```python
from build123d import *

# Parameters (mm, degrees)
BOX138_W     = 17
BOX138_H     = 24
BOX138_DEPTH = 11
BOX137_W     = 43
BOX137_H     = 27
BOX137_DEPTH = 11
BOX136_W     = 50
BOX136_H     = 37
BOX136_DEPTH = 13
BOX135_W     = 55
BOX135_H     = 40
BOX135_DEPTH = 16


with BuildPart() as cube060:
    # Box138 → Box138 (new body)
    with BuildSketch(Plane(origin=(337.5, 106, 176), x_dir=(1, 0, 0), z_dir=(0, 0, -1))):
        with Locations((8.5, 12)):
            Rectangle(BOX138_W, BOX138_H)
    extrude(amount=BOX138_DEPTH)


with BuildPart() as cube059:
    # Box137 → Box137 (new body)
    with BuildSketch(Plane(origin=(345.5, 111, 185), x_dir=(1, 0, 0), z_dir=(0, 0, -1))):
        with Locations((21.5, 13.5)):
            Rectangle(BOX137_W, BOX137_H)
    extrude(amount=BOX137_DEPTH)


with BuildPart() as cube058:
    # Box136 → Box136 (new body)
    with BuildSketch(Plane(origin=(342, 121, 181.5), x_dir=(1, 0, 0), z_dir=(0, 0, -1))):
        with Locations((25, 18.5)):
            Rectangle(BOX136_W, BOX136_H)
    extrude(amount=BOX136_DEPTH)


with BuildPart() as cut026:
    # Box135 → Box135 (new body)
    with BuildSketch(Plane(origin=(340, 124, 183), x_dir=(1, 0, 0), z_dir=(0, 0, -1))):
        with Locations((27.5, 20)):
            Rectangle(BOX135_W, BOX135_H)
    extrude(amount=BOX135_DEPTH)

    # Cut024: cut Cube058
    add(cube058.part, mode=Mode.SUBTRACT)

    # Cut025: cut Cube059
    add(cube059.part, mode=Mode.SUBTRACT)

    # Cut026: cut Cube060
    add(cube060.part, mode=Mode.SUBTRACT)


solid = cut026.part
```
Model file for the job. Use its own axes, mm. A direction names the side the tool comes from. Round coordinates to 2 decimals unless told otherwise and drop trailing zeros. Write each loop counter-clockwise with the first axis right and the second up, starting at its lowest first coordinate (ties: lowest second). Pieces come first, ordered by that corner, then holes. Notation, with made-up numbers: (77, 27.5) -> (122, 27.5) arc R26 ccw to (122, 49.5) -> close; hole circle Ø10 at (-15.75, 63.25). An arc over 180 degrees is marked (long way). Answer as CSV lines item,"result".
1. Slice it at D-D, the plane y = 113. List the corners of the cut face in (x, z), plus the area to 3 significant figures.
Resolved:
outline,"(340, 167) -> (395, 167) -> (395, 183) -> (340, 183) -> close; hole (342, 168.5) -> (392, 168.5) -> (392, 181.5) -> (342, 181.5) -> close"
area,"230 mm²"
2. Mould opens along X. For faces 4 (the face through (367, 102, 168.5)), 5 (the face through (354.5, 95, 168)), 6 (the face through (367, 113, 183)) say: +X half, -X half, draft (parallel to the pull), parting line (faces both ways), or undercut.
Resolved:
face 4,"undercut"
face 5,"-X half"
face 6,"draft"
3. Drill centre lines: line 1 (X direction, y = 115, z = 180); line 2 (Z direction, x = 379, y = 117.5); line 3 (Z direction, x = 360.5, y = 87). Where is each one in solid material? Low to high.
Resolved:
line 1,"340 to 342, 392 to 395"
line 2,"167 to 168.5, 181.5 to 183"
line 3,"167 to 168.5"
4. Slice it at C-C, the plane x = 383. List the corners of the cut face in (y, z), plus the area to 4 significant figures.
Resolved:
outline,"(84, 167) -> (124, 167) -> (124, 183) -> (111, 183) -> (111, 181.5) -> (121, 181.5) -> (121, 168.5) -> (84, 168.5) -> close"
area,"118.5 mm²"
5. Pin check, flat tips, straight feed: pin 1 Ø1.2 at (x, z) = (357.5, 182.5) entering from -Y; pin 2 Ø1 at (x, z) = (357, 180.5) entering from -Y; pin 3 Ø2 at (x, y) = (341, 91) entering from -Z. Stop position of each tip, or through.
Resolved:
pin 1,"y = 111"
pin 2,"y = 121"
pin 3,"z = 176"
6. Slice it at A-A, the plane y = 96. List the corners of the cut face in (x, z), plus the area to 3 significant figures.
Resolved:
outline,"(340, 176) -> (342, 176) -> (342, 181.5) -> (345.5, 181.5) -> (345.5, 183) -> (340, 183) -> close; (354.5, 167) -> (395, 167) -> (395, 183) -> (388.5, 183) -> (388.5, 181.5) -> (392, 181.5) -> (392, 168.5) -> (354.5, 168.5) -> close"
area,"129 mm²"
7. Tool access for faces 1 (the face through (367, 121, 175)), 2 (the face through (345.5, 98, 182)), 3 (the face through (345, 106, 168)): list every direction of +Z, -Z, +X, -X, +Y, -Y with a clear straight run to the whole face (end or side of a thin tool).
Resolved:
face 1,"-Y"
face 2,"+Z, -Y"
face 3,"-Z, -X, -Y"
8. Slice it at B-B, the plane z = 177.25. List the corners of the cut face in (x, y), plus the area to 3 significant figures.
Resolved:
outline,"(340, 84) -> (342, 84) -> (342, 121) -> (392, 121) -> (392, 84) -> (395, 84) -> (395, 124) -> (340, 124) -> close"
area,"350 mm²"
